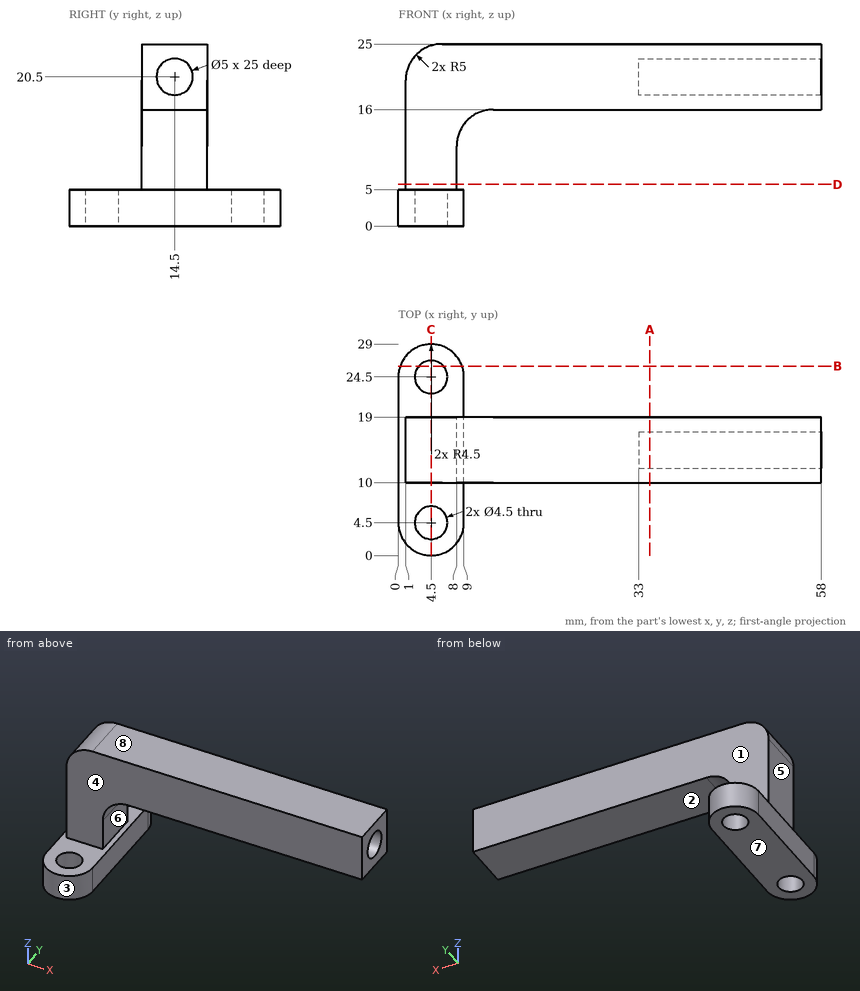
Could you check a few things on this drawing? It's one solid part, dimensions in mm from its lowest x, y, z. A direction names the side the tool comes from. Round coordinates to 2 decimals unless told otherwise and drop trailing zeros. Order: outer loops, then holes, each group sorted by start corner. A loop starts at its lowest first (then second) coordinate and runs counter-clockwise, first axis right, second up.
Q1. Please list where these lines run through material, in increasing order: probe 1 along Y at (x, z) = (4.5, 2.65); probe 2 along Y at (x, z) = (51, 20.5); probe 3 along X at (y, z) = (3.5, 4).
Geometry says:
probe 1: y = 0 to 2.25, 6.75 to 22.25, 26.75 to 29
probe 2: y = 10 to 12, 17 to 19
probe 3: x = 0.11 to 2.48, 6.52 to 8.89
Q2. Thinking about a two-plate mould opening in Z: for the marked faces 5, 6, 7 and 8, which applies, released by +Z, released by -Z, zero draft, split by the parting line, or undercut?
Geometry says:
face 5: zero draft
face 6: undercut
face 7: released by -Z
face 8: released by +Z
Q3. Imagine slicing it at A-A, the plane x = 34.5. List the corners of the cut face in (y, z) for me.
Geometry says:
outline: (10, 16) - (19, 16) - (19, 25) - (10, 25) - close; hole circle Ø5 at (14.5, 20.5)
Q4. Imagine slicing it at B-B, the plane y = 26. List the corners of the cut face in (x, z) for me.
Geometry says:
outline: (0.26, 0) - (2.82, 0) - (2.82, 5) - (0.26, 5) - close; (6.18, 0) - (8.74, 0) - (8.74, 5) - (6.18, 5) - close
Q5. Imagine slicing it at D-D, the plane z = 5.75. List the corners of the cut face in (x, y) for me.
Geometry says:
outline: (1, 10) - (8, 10) - (8, 19) - (1, 19) - close
Q6. I'm going to push flat-ended pins straight in: P1, Ø4.5, axis at y = 14.5, z = 20.5, coming from the +X side; P2, Ø12, axis at y = 16, z = 9, coming from the +X side; P3, Ø3, axis at y = 12.5, z = 9, coming from the +X side. Where does each tip first touch, or does it pass through?
Geometry says:
P1: stops at x = 33
P2: stops at x = 10
P3: stops at x = 8
Q7. Imagine slicing it at C-C, the plane x = 4.5. List the corners of the cut face in (y, z) for me.
Geometry says:
outline: (0, 0) - (2.25, 0) - (2.25, 5) - (0, 5) - close; (6.75, 0) - (22.25, 0) - (22.25, 5) - (19, 5) - (19, 24.77) - (10, 24.77) - (10, 5) - (6.75, 5) - close; (26.75, 0) - (29, 0) - (29, 5) - (26.75, 5) - close
Q8. Which directions (+Z, -Z, +X, -X, +Y, -Y) give clear straight access to the entire face, cutting with the end or side of a thin tool? Please do the marked faces 1, 2, 3 and 4.
Geometry says:
face 1: +Z, +X, -X, +Y
face 2: -Z, +X, +Y, -Y
face 3: +Z, -Z, -Y
face 4: +Z, +X, -X, -Y
